The drawing under review shows one solid part. Ordinate dimensions are in mm from its lowest x, y, z. A direction names the side the tool comes from. Give positions to 0.01 mm unless a question says otherwise; leave off trailing zeros. Write each loop counter-clockwise with the first axis right and the second up, starting at its lowest first coordinate (ties: lowest second). Pieces come first, ordered by that corner, then holes. Notation, with made-up numbers: (40.5, 59) - (75.5, 59) arc R21 ccw to (75.5, 65) - close; hole circle Ø10 at (82.5, -4). An arc over 180 degrees is marked (long way). Write item = value, one per line.
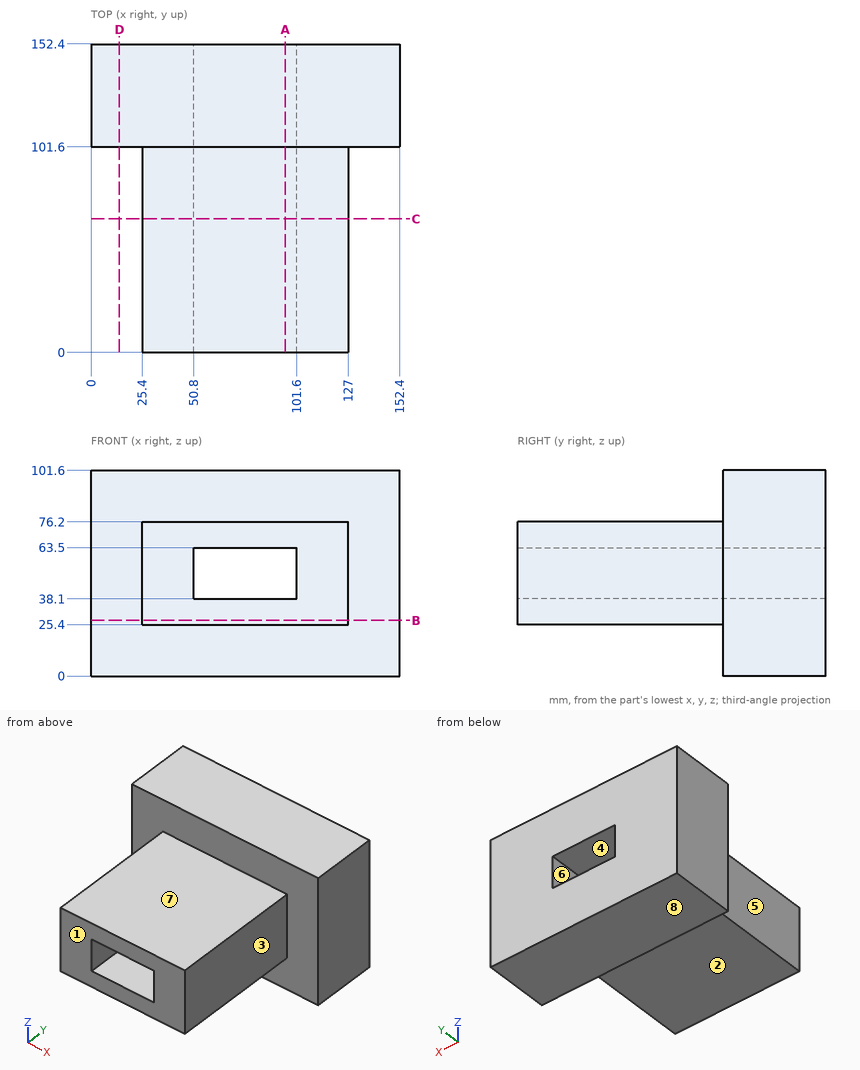
1. Take a section at D-D on x = 14. Give the boundary of the cut face in (y, z).
Findings below:
outline = (101.6, 0) - (152.4, 0) - (152.4, 101.6) - (101.6, 101.6) - close
2. Insertion check: P1, Ø3, axis at y = 78, z = 47, coming from the -X side; P2, Ø3, axis at y = 136.5, z = 64, coming from the -X side; P3, Ø1, axis at y = 24.5, z = 25.5, coming from the +X side; P4, Ø2, axis at x = 46.5, y = 65, coming from the +Z side. Each pin has a flat end and moves straight along its axis. Give the tip position at first contact, or say it passes through.
Findings below:
P1 = 25.4
P2 = 0
P3 = 127
P4 = 76.2
3. Machinability: for the marked faces 1, 2, 3, 4 and 5, which of the approach directions +Z, -Z, +X, -X, +Y, -Y give a long, thin tool a straight path to every point of the face, cutting with its end or side? Answer none if there is none.
Findings below:
face_1 = +Z, -Z, +X, -X, -Y
face_2 = -Z, +X, -X, -Y
face_3 = +Z, -Z, +X, -Y
face_4 = +Y, -Y
face_5 = +Z, -Z, -X, -Y
4. Draft analysis for pull direction Z (two halves, no side actions). For the marked faces 6, 7 and 8, state which applies: +Z half, -Z half, draft (parallel to the pull), parting line (faces both ways), or undercut.
Findings below:
face_6 = undercut
face_7 = +Z half
face_8 = -Z half
5. For line 1 (X direction, y = 40, z = 45.5); line 2 (X direction, y = 104.5, z = 51); line 3 (Z direction, x = 99, y = 17.5), list the stretches that pass through material, from the lowest coordinate up. Write a range as from..to.
Findings below:
line_1 = 25.4..50.8, 101.6..127
line_2 = 0..50.8, 101.6..152.4
line_3 = 25.4..38.1, 63.5..76.2
6. Take a section at A-A on x = 96. Give the boundary of the cut face in (y, z), and give its area (3 significant figures).
Findings below:
outline = (0, 25.4) - (101.6, 25.4) - (101.6, 0) - (152.4, 0) - (152.4, 38.1) - (0, 38.1) - close; (0, 63.5) - (152.4, 63.5) - (152.4, 101.6) - (101.6, 101.6) - (101.6, 76.2) - (0, 76.2) - close
area = 6,450 mm²
7. Take a section at B-B on z = 27.5. Give the boundary of the cut face in (x, y), and give its area (3 significant figures).
Findings below:
outline = (0, 101.6) - (25.4, 101.6) - (25.4, 0) - (127, 0) - (127, 101.6) - (152.4, 101.6) - (152.4, 152.4) - (0, 152.4) - close
area = 18,100 mm²
8. Take a section at C-C on y = 66. Give the boundary of the cut face in (x, z).
Findings below:
outline = (25.4, 25.4) - (127, 25.4) - (127, 76.2) - (25.4, 76.2) - close; hole (50.8, 38.1) - (101.6, 38.1) - (101.6, 63.5) - (50.8, 63.5) - close
